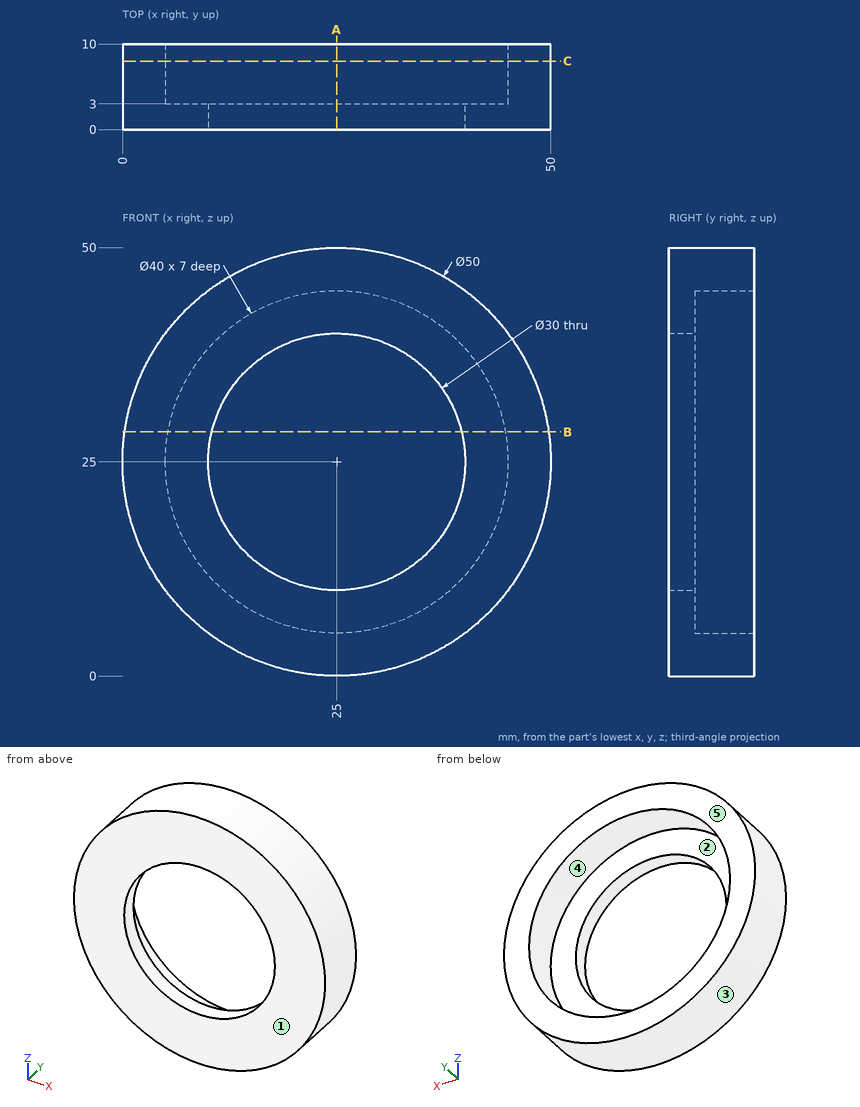
For this review, use the dimensioned drawing (mm, ordinates from the lowest corner) and the shaded views. A direction names the side the tool comes from. Round coordinates to 2 decimals unless told otherwise and drop trailing zeros. Loops run counter-clockwise (first coordinate to the right, second up) from the corner with the lowest first, then second, coordinate; pieces in that order, holes last. Notation, with made-up numbers: (49.5, 54.25) -> (71.5, 54.25) arc R10 ccw to (71.5, 60.25) -> close; hole circle Ø7 at (56.5, 83). An arc over 180 degrees is marked (long way). Write item = value, one per line. Start each with the question number.
Item 1: To check wall thickness, follow L1, parallel to Z at x = 25, y = 1.6; L2, parallel to Z at x = 25, y = 5.5; L3, parallel to X at y = 9, z = 39. State the ranges of each line that lie inside material, in increasing order.
Item 2: Take a section at C-C on y = 8. Give the boundary of the cut face in (x, z).
Item 3: Take a section at B-B on z = 28.5. Give the boundary of the cut face in (x, y), plus the area to 3 significant figures.
Item 4: Insertion check: pin 1 (1 mm diameter, centred on y = 6, z = 24, fed in from +X) (3 decimals); pin 2 (3 mm diameter, centred on y = 4.5, z = 42, fed in from +X); pin 3 (1 mm diameter, centred on x = 39.5, y = 1.5, fed in from +Z). Each pin has a flat end and moves straight along its axis. Give the tip position at first contact, or say it passes through.
Item 5: Mouldability with a two-part tool opening along X and no side actions: class the marked faces 3, 4 and 5 as released by +X, released by -X, zero draft, split by the parting line, or undercut.
Item 6: For the marked faces 1 and 2, list the 3-axis set-ups (+Z, -Z, +X, -X, +Y, -Y) from which the entire face can be reached by the end or side of a thin tool; tool diameter is ignored.
Item 7: Take a section at A-A on x = 25. Give the boundary of the cut face in (y, z).
Result:
q1.L1 = 0 to 10, 40 to 50
q1.L2 = 0 to 5, 45 to 50
q1.L3 = 4.29 to 10.72, 39.28 to 45.71
q2.outline = circle Ø50 at (25, 25); hole circle Ø40 at (25, 25)
q3.outline = (0.25, 0) -> (10.41, 0) -> (10.41, 3) -> (5.31, 3) -> (5.31, 10) -> (0.25, 10) -> close; (39.59, 0) -> (49.75, 0) -> (49.75, 10) -> (44.69, 10) -> (44.69, 3) -> (39.59, 3) -> close
q3.area = 132 mm²
q4.pin_1 = 49.995
q4.pin_2 = 44.62
q4.pin_3 = 45.71
q5.face_3 = split by the parting line
q5.face_4 = undercut
q5.face_5 = zero draft
q6.face_1 = +Z, -Z, +X, -X, -Y
q6.face_2 = +Y
q7.outline = (0, 0) -> (10, 0) -> (10, 5) -> (3, 5) -> (3, 10) -> (0, 10) -> close; (0, 40) -> (3, 40) -> (3, 45) -> (10, 45) -> (10, 50) -> (0, 50) -> close
